from build123d import *

# Parameters (mm, degrees)
SKETCH1_R              = 15.55
BACK_DEPTH             = 42.5
SKETCH3_R              = 17.6
FRONT_DEPTH            = 18
SKETCH4_R              = 6
SHAFTBEARING_DEPTH     = 1.8
SKETCH5_R              = 1.75
FRONTSCREWHOLES_DEPTH  = 5.5
SKETCH6_R              = 2.5
ROUNDPARTOFSHAFT_DEPTH = 1.2
FLATPARTOFSHAFT_DEPTH  = 9.5
SKETCH8_RX             = 2.553008369
SKETCH8_RY             = 1.011966428
PWR_AND_GND_DEPTH      = 7


with BuildPart() as part:
    # Sketch1 → Back (new body)
    with BuildSketch(Plane.XY):
        Circle(SKETCH1_R)
    extrude(amount=-BACK_DEPTH)

    # Sketch3 → Front (add)
    with BuildSketch(Plane.XY):
        Circle(SKETCH3_R)
    extrude(amount=FRONT_DEPTH)

    # Sketch4 → ShaftBearing (add)
    with BuildSketch(Plane.XY.offset(18)):
        with Locations((0, -8.73)):
            Circle(SKETCH4_R)
    extrude(amount=SHAFTBEARING_DEPTH)

    # Sketch5 → frontScrewHoles (cut)
    with BuildSketch(Plane.XY.offset(18)):
        with Locations((-10.25, -8.73)):
            Circle(SKETCH5_R)
        with Locations((10.250000074, -8.73)):
            Circle(SKETCH5_R)
        with Locations((0, 13.37)):
            Circle(SKETCH5_R)
    extrude(amount=-FRONTSCREWHOLES_DEPTH, mode=Mode.SUBTRACT)

    # Sketch6 → RoundPartofShaft (add)
    with BuildSketch(Plane.XY.offset(19.8)):
        with Locations((0, -8.73)):
            Circle(SKETCH6_R)
    extrude(amount=ROUNDPARTOFSHAFT_DEPTH)

    # Sketch7 → FlatPartofShaft (add)
    with BuildSketch(Plane.XY.offset(21)):
        with BuildLine():
            Line((2, -7.23), (-2, -7.23))
            ThreePointArc((-2, -7.23), (0, -11.23), (2, -7.23))
        make_face()
    extrude(amount=FLATPARTOFSHAFT_DEPTH)

    # Sketch8 → Pwr And Gnd (add)
    with BuildSketch(Plane(origin=(0, 0, -42.5), x_dir=(-1, 0, 0), z_dir=(0, 0, -1))):
        with Locations(Location((9.443035065, -4.815505038), (0, 0, -117.019449203))):
            Ellipse(SKETCH8_RX, SKETCH8_RY)
        with Locations(Location((-9.44630216, 4.809093002), (0, 0, 63.019449203))):
            Ellipse(SKETCH8_RX, SKETCH8_RY)
    extrude(amount=PWR_AND_GND_DEPTH)


solid = part.part
Can you work these out from the model? Positions are in its coordinate system, mm. A direction names the side the tool comes from. Coordinates: 2 decimals unless noted, no trailing zeros. Loops run counter-clockwise (first coordinate to the right, second up) from the corner with the lowest first, then second, coordinate; pieces in that order, holes last. Notation, with made-up numbers: M 62,45.5 L 99,45.5 A23 cw 99,57.5 Z; hole C 20.5,46 d2. An arc over 180 degrees is marked long. Answer as CSV lines item,"result". Start each with the question number.
1. Suppose I cut it at C-C, the plane z = -8.5. List the corners of the cut face in (x, y) for me.
2. If I drill on probe 1 along Y at (x, z) = (0, 16.5); probe 2 along Z at (x, y) = (-1.5, -5.5); probe 3 along X at (y, z) = (13, 16), over which ranges is the centre line in solid material (lowest first)? Write a range as [from, to].
3. For faces 1 (the face through (0, -7.23, 26)), 2 (the face through (-3.37, -15.18, -20.95)), 3 (the face through (-0.78, -2.78, 18.89)), which set-ups out of +Z, -Z, +X, -X, +Y, -Y let a thin tool reach every point of the face, with its end or its side?
4. Suppose I cut it at D-D, the plane x = 14. List the corners of the cut face in (y, z) for me.
5. Suppose I cut it at A-A, the plane x = 0. List the corners of the cut face in (y, z) for me.
6. Suppose I cut it at B-B, the plane y = 0. List the corners of the cut face in (x, z) for me.
7. For pin 1 Ø3 at (x, y) = (10.5, 0) entering from -Z; pin 2 Ø3 at (x, y) = (0, 13.37) entering from +Z; pin 3 Ø1.1 at (x, y) = (0, -6.5) entering from +Z; pin 4 Ø1.5 at (x, y) = (-13, -13.5) entering from +Z, each with a flat end and sliding along its axis, tell me the tip position at first contact or that it passes through.
8. Thinking about a two-plate mould opening in Y: for faces 4 (the face through (0, 13, 12.5)), 5 (the face through (16.787, 5.287, 8.874)), 6 (the face through (0, 0, 18)), which applies, +Y half, -Y half, draft (parallel to the pull), parting line (faces both ways), or undercut?
Output:
1,outline,"C 0,0 d31.1"
2,probe 1,"y = [-17.6, 11.62], [15.12, 17.6]"
2,probe 2,"z = [-42.5, 19.8]"
2,probe 3,"x = [-11.86, -1.71], [1.71, 11.86]"
3,face 1,"+Z, +X, -X, +Y"
3,face 2,"-Z"
3,face 3,"+Z"
4,outline,"M -10.67,0 L -6.77,0 L -6.77,-42.5 L 6.77,-42.5 L 6.77,0 L 10.67,0 L 10.67,18 L -10.67,18 Z"
5,outline,"M -17.6,0 L -15.55,0 L -15.55,-42.5 L 15.55,-42.5 L 15.55,0 L 17.6,0 L 17.6,18 L 15.12,18 L 15.12,12.5 L 11.62,12.5 L 11.62,18 L -2.73,18 L -2.73,19.8 L -6.23,19.8 L -6.23,21 L -7.23,21 L -7.23,30.5 L -11.23,30.5 L -11.23,19.8 L -14.73,19.8 L -14.73,18 L -17.6,18 Z"
6,outline,"M -17.6,0 L -15.55,0 L -15.55,-42.5 L 15.55,-42.5 L 15.55,0 L 17.6,0 L 17.6,18 L -17.6,18 Z"
7,pin 1,"stops at z = -42.5"
7,pin 2,"stops at z = 12.5"
7,pin 3,"stops at z = 21"
7,pin 4,"passes through"
8,face 4,"undercut"
8,face 5,"parting line"
8,face 6,"draft"
